Input: dimensioned drawing with shaded views. Units: mm. Origin: part minimum x, y, z. A direction names the side the tool comes from. Give positions to 0.01 mm unless a question says otherwise; leave off trailing zeros. Write each loop counter-clockwise with the first axis right and the second up, starting at its lowest first coordinate (ties: lowest second). Pieces come first, ordered by that corner, then holes.
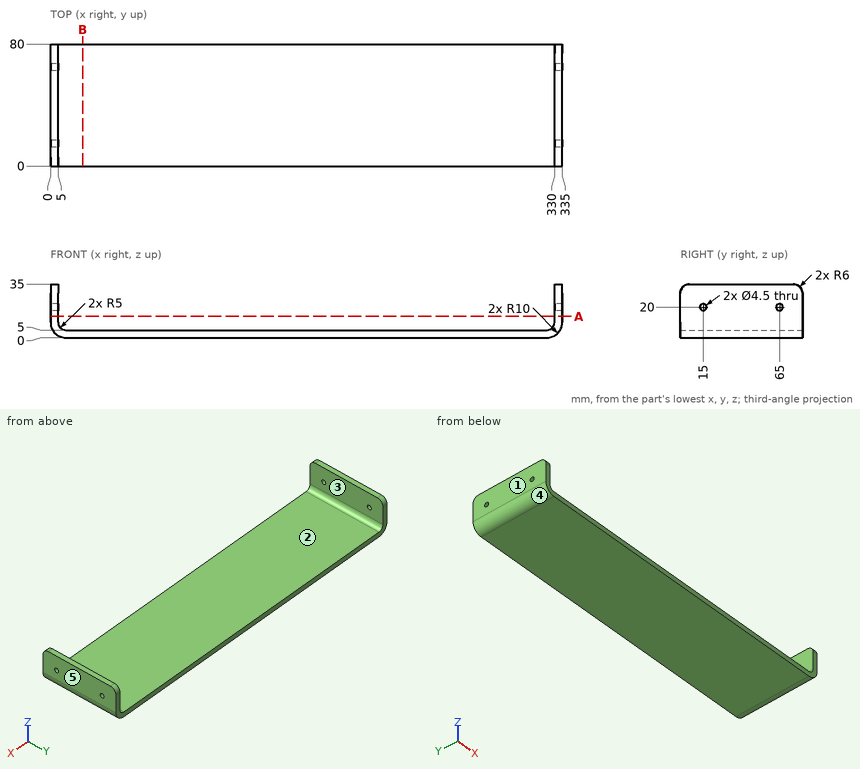
Item 1: Section B-B, the plane x = 21. Return the cut outline in (y, z).
Found:
outline: (0, 0) - (80, 0) - (80, 5) - (0, 5) - close
Item 2: Pin query (flat end, axial travel): pin 1 Ø5 at (x, y) = (121, 41.5) entering from +Z. Return the tip coordinate at first contact, or that it passes through.
Found:
pin 1: stops at z = 5
Item 3: Section A-A, the plane z = 14. Return the cut outline in (x, y).
Found:
outline: (0, 0) - (5, 0) - (5, 80) - (0, 80) - close; (330, 0) - (335, 0) - (335, 80) - (330, 80) - close
Item 4: Line query: L1, parallel to Y at x = 332, z = 20; L2, parallel to X at y = 18, z = 19; L3, parallel to Z at x = 253.5, y = 76.5. Output: solid intervals per line, ascending.
Found:
L1: y = 0 to 12.75, 17.25 to 62.75, 67.25 to 80
L2: x = 0 to 5, 330 to 335
L3: z = 0 to 5
Item 5: Pull-direction query (X, two-part tool) for the marked faces 3, 4 and 5; classes: +X half, -X half, draft (parallel to the pull), parting line (faces both ways), or undercut.
Found:
face 3: undercut
face 4: -X half
face 5: +X half
Item 6: Reachability of the marked faces 1 and 2 from +Z, -Z, +X, -X, +Y, -Y: full face, straight path, thin tool, end or side. Return the list, or none.
Found:
face 1: +Z, -Z, -X, +Y, -Y
face 2: +Z, +Y, -Y
